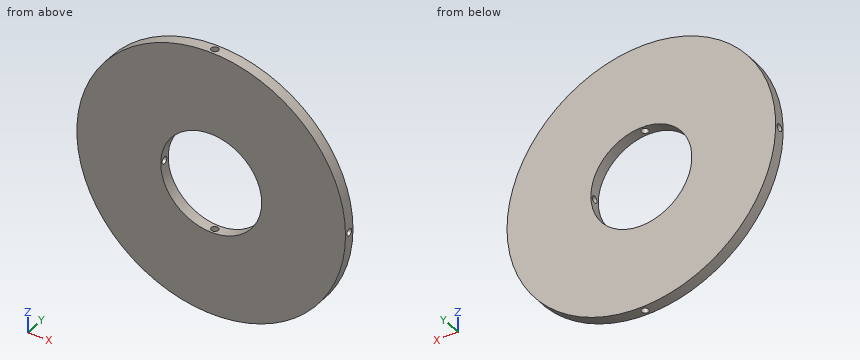
```python
from build123d import *

# Parameters (mm, degrees)
F0_R     = 76.2
F0_R_2   = 28.6385
F1_DEPTH = 6.35
F4_D     = 4.0386
F7_D     = 4.0386


# Not quite as in the source:
# - a feature names something its author has since deleted; it is built from what else it names


with BuildPart() as f1:
    # F0 (on Front) → F1 (new body)
    with BuildSketch(Plane.XZ):
        Circle(F0_R)
        Circle(F0_R_2, mode=Mode.SUBTRACT)
    extrude(amount=F1_DEPTH)

    # F4 (through all)
    with Locations(Plane.XY.offset(76.2)):
        with Locations((0, -3.175)):
            Hole(F4_D / 2)

    # F7 (through all)
    with Locations(Plane.YZ.offset(76.2)):
        with Locations((-3.175, 0)):
            Hole(F7_D / 2)


solid = f1.part
```
Source: CAD feature listing. Evaluate the final solid. Frame: model axes, mm. Round coordinates to 2 decimals unless told otherwise and drop trailing zeros. Loops run counter-clockwise (first coordinate to the right, second up) from the corner with the lowest first, then second, coordinate; pieces in that order, holes last. Notation, with made-up numbers: M 43,25 L 69,25 A18 cw 69,55 Z; hole C 46.5,-32.5 d6. An arc over 180 degrees is marked long. Use a Markdown table: item, result. Add a question column.
1. Contact query for a flat-ended pin moving along its axis: P1, Ø3, axis at y = -3.175, z = 0, coming from the -X side. Output: stop coordinate, or through.
2. Line query: line 1 (Y direction, x = 0, z = 55); line 2 (X direction, y = -5, z = 57); line 3 (Z direction, x = 46, y = -3.75). Output: solid intervals per line, ascending.
3. Section query D-D on z = 39. Return the cut outline in (x, y) (3 decimals), then the cut area to 3 significant figures.
4. Section query A-A on z = 0. Return the cut outline in (x, y).
5. Section query B-B on x = 0. Return the cut outline in (y, z), then the cut area to 3 significant figures.
6. Section query C-C on x = -22.5. Return the cut outline in (y, z).
Reported:
| question | item | result |
|---|---|---|
| 1 | P1 | passes through |
| 2 | line 1 | y = -6.35 to -5.19, -1.16 to 0 |
| 2 | line 2 | x = -50.57 to -0.86, 0.86 to 50.57 |
| 2 | line 3 | z = -60.75 to -1.94, 1.94 to 60.75 |
| 3 | outline | M -65.463,-6.35 L 65.463,-6.35 L 65.463,0 L -65.463,0 Z; hole C 0,-3.175 d4.039 |
| 3 | area | 819 mm² |
| 4 | outline | M -76.2,-6.35 L -28.64,-6.35 L -28.64,-5.19 L -76.2,-5.19 Z; M -76.2,-1.16 L -28.64,-1.16 L -28.64,0 L -76.2,0 Z; M 28.64,-6.35 L 76.2,-6.35 L 76.2,-5.19 L 28.64,-5.19 Z; M 28.64,-1.16 L 76.2,-1.16 L 76.2,0 L 28.64,0 Z |
| 5 | outline | M -6.35,-76.2 L -5.19,-76.2 L -5.19,-28.64 L -6.35,-28.64 Z; M -6.35,28.64 L -5.19,28.64 L -5.19,76.2 L -6.35,76.2 Z; M -1.16,-76.2 L 0,-76.2 L 0,-28.64 L -1.16,-28.64 Z; M -1.16,28.64 L 0,28.64 L 0,76.2 L -1.16,76.2 Z |
| 5 | area | 220 mm² |
| 6 | outline | M -6.35,-72.8 L 0,-72.8 L 0,-17.72 L -6.35,-17.72 Z; M -6.35,17.72 L 0,17.72 L 0,72.8 L -6.35,72.8 Z |
